```python
from build123d import *

# Parameters (mm, degrees)
SKETCH1_W           = 184.64
SKETCH1_H           = 137
SKETCH1_R           = 3.65
SKETCH1_R_2         = 3.57
SKETCH1_R_3         = 2.5
BOSS_EXTRUDE1_DEPTH = 4
SKETCH3_W           = 104.64
SKETCH3_H           = 20
BOSS_EXTRUDE2_DEPTH = 4
SKETCH6_R           = 3.65
CUT_EXTRUDE4_DEPTH  = 5
SKETCH8_W           = 140
SKETCH8_H           = 16
CUT_EXTRUDE6_DEPTH  = 10
FILLET5_R           = 2
SKETCH11_W          = 184.64
SKETCH11_H          = 15
SKETCH11_R          = 2.5
BOSS_EXTRUDE4_DEPTH = 4
SKETCH12_R          = 2.5
CUT_EXTRUDE8_DEPTH  = 5
SKETCH13_R          = 2.5
CUT_EXTRUDE9_DEPTH  = 10
SKETCH14_W          = 1.5
SKETCH14_H          = 3
CUT_EXTRUDE10_DEPTH = 5


with BuildPart() as part:
    # Sketch1 → Boss-Extrude1 (new body)
    with BuildSketch(Plane.XY):
        with Locations((92.32, 68.5)):
            Rectangle(SKETCH1_W, SKETCH1_H)
        with Locations((15, 16)):
            Circle(SKETCH1_R, mode=Mode.SUBTRACT)
        with Locations((169.64, 16)):
            Circle(SKETCH1_R, mode=Mode.SUBTRACT)
        with Locations((15, 121)):
            Circle(SKETCH1_R_2, mode=Mode.SUBTRACT)
        with Locations((30, 96)):
            Circle(SKETCH1_R_3, mode=Mode.SUBTRACT)
        with Locations((169.64, 121)):
            Circle(SKETCH1_R_2, mode=Mode.SUBTRACT)
        with Locations((154.64, 96)):
            Circle(SKETCH1_R_3, mode=Mode.SUBTRACT)
        Polygon((40, 106), (40, 86), (22.32, 86), (22.32, 56), (162.32, 56), (162.32, 86), (144.64, 86), (144.64, 106), align=None, mode=Mode.SUBTRACT)
    extrude(amount=BOSS_EXTRUDE1_DEPTH)

    # Sketch3 → Boss-Extrude2 (add)
    with BuildSketch(Plane.XY.offset(4)):
        with Locations((92.32, 96)):
            Rectangle(SKETCH3_W, SKETCH3_H)
    extrude(amount=-BOSS_EXTRUDE2_DEPTH)

    # Sketch6 → Cut-Extrude4 (cut, through all)
    with BuildSketch(Plane.XY.offset(4)):
        with Locations((67.32, 16)):
            Circle(SKETCH6_R)
        with Locations((117.32, 16)):
            Circle(SKETCH6_R)
    extrude(amount=-CUT_EXTRUDE4_DEPTH, mode=Mode.SUBTRACT)

    # Sketch8 → Cut-Extrude6 (cut)
    with BuildSketch(Plane.XY.offset(4)):
        with Locations((92.32, 48)):
            Rectangle(SKETCH8_W, SKETCH8_H)
    extrude(amount=-CUT_EXTRUDE6_DEPTH, mode=Mode.SUBTRACT)

    # Fillet5
    fillet5_edges = [part.edges().sort_by_distance(p)[0] for p in [
        (0, 137, 2),
        (184.64, 137, 2),
        (184.64, 0, 2),
        (0, 0, 2),
    ]]
    fillet(fillet5_edges, radius=FILLET5_R)

    # Sketch11 → Boss-Extrude4 (add, through all)
    with BuildSketch(Plane.XY.offset(4)):
        with Locations((92.32, 16)):
            Rectangle(SKETCH11_W, SKETCH11_H)
        with Locations((15, 16)):
            Circle(SKETCH11_R, mode=Mode.SUBTRACT)
        with Locations((169.64, 16)):
            Circle(SKETCH11_R, mode=Mode.SUBTRACT)
    extrude(amount=-BOSS_EXTRUDE4_DEPTH)

    # Sketch12 → Cut-Extrude8 (cut, through all)
    with BuildSketch(Plane.XY.offset(4)):
        with Locations((10, 96)):
            Circle(SKETCH12_R)
        with Locations((174.64, 96)):
            Circle(SKETCH12_R)
    extrude(amount=-CUT_EXTRUDE8_DEPTH, mode=Mode.SUBTRACT)

    # Sketch13 → Cut-Extrude9 (cut)
    with BuildSketch(Plane.XY.offset(4)):
        with Locations((173.48, 67)):
            Circle(SKETCH13_R)
    extrude(amount=-CUT_EXTRUDE9_DEPTH, mode=Mode.SUBTRACT)

    # Sketch14 → Cut-Extrude10 (cut, through all)
    with BuildSketch(Plane.XY.offset(4)):
        with Locations((171.48, 59)):
            Rectangle(SKETCH14_W, SKETCH14_H)
        with Locations((175.48, 59)):
            Rectangle(SKETCH14_W, SKETCH14_H)
    extrude(amount=-CUT_EXTRUDE10_DEPTH, mode=Mode.SUBTRACT)


solid = part.part
```
Build history of the part. All positions in model axes, mm. A direction names the side the tool comes from. Coordinates: 2 decimals unless noted, no trailing zeros. Order: outer loops, then holes, each group sorted by start corner. A loop starts at its lowest first (then second) coordinate and runs counter-clockwise, first axis right, second up. Notation, with made-up numbers: (77.25, 13.25) -> (107.25, 13.25) arc R19 cw to (107.25, 42.25) -> close; hole circle Ø9 at (-9.5, -39.75). An arc over 180 degrees is marked (long way). Answer in a Markdown table with one row per item. Add a question column.
Q1. Band-saw the part on B-B, the plane x = 154.64. List the corners of the cut face in (y, z).
Q2. Drop flat-ended pins along their axis: pin 1 (8 mm diameter, centred on x = 15, y = 121, fed in from +Z); pin 2 (4 mm diameter, centred on x = 169.64, y = 16, fed in from -Z). Give the stop position or say it passes through.
Q3. Band-saw the part on C-C, the plane y = 47.5. List the corners of the cut face in (x, z).
Q4. Wall check: line 1 along X through (y, z) = (58, 1.3); line 2 along Y through (x, z) = (15, 2.6); line 3 along Y through (x, z) = (102.5, 0.2). Give the ranges that are in metal, low to high. Write a range as [from, to].
Q5. Mould opens along X. For faces 1 (the face through (9.67, 98.48, 2.03)), 2 (the face through (172.142, 96.11, 2.028)), 3 (the face through (184.64, 68, 2)), 4 (the face through (0, 68, 2)) say: +X half, -X half, draft (parallel to the pull), parting line (faces both ways), or undercut.
Q6. Band-saw the part on A-A, the plane y = 16. List the corners of the cut face in (x, z).
Q7. Band-saw the part on D-D, the plane z = 1.8. Give the number of separate pieces and of enclosed holes in the cut face, then the cut area to 3 significant figures.
Q8. Which spindle directions (+Z, -Z, +X, -X, +Y, -Y) get a long thin tool onto all of the face, cutting with end or side? Do faces 5 (the face through (91, 40, 2)), 6 (the face through (91, 0, 2)). Say none if no direction does.
Answers follow:
| question | item | result |
|---|---|---|
| 1 | outline | (0, 0) -> (40, 0) -> (40, 4) -> (0, 4) -> close; (86, 0) -> (93.5, 0) -> (93.5, 4) -> (86, 4) -> close; (98.5, 0) -> (137, 0) -> (137, 4) -> (98.5, 4) -> close |
| 2 | pin 1 | z = 4 |
| 2 | pin 2 | through |
| 3 | outline | (0, 0) -> (22.32, 0) -> (22.32, 4) -> (0, 4) -> close; (162.32, 0) -> (184.64, 0) -> (184.64, 4) -> (162.32, 4) -> close |
| 4 | line 1 | [0, 22.32], [162.32, 170.73], [172.23, 174.73], [176.23, 184.64] |
| 4 | line 2 | [0, 13.5], [18.5, 117.43], [124.57, 137] |
| 4 | line 3 | [0, 40], [86, 137] |
| 5 | face 1 | undercut |
| 5 | face 2 | undercut |
| 5 | face 3 | +X half |
| 5 | face 4 | -X half |
| 6 | outline | (0, 0) -> (12.5, 0) -> (12.5, 4) -> (0, 4) -> close; (17.5, 0) -> (167.14, 0) -> (167.14, 4) -> (17.5, 4) -> close; (172.14, 0) -> (184.64, 0) -> (184.64, 4) -> (172.14, 4) -> close |
| 7 | separate pieces | 1 |
| 7 | enclosed holes | 12 |
| 7 | area | 18,600 mm^2 |
| 8 | face 5 | +Z, -Z |
| 8 | face 6 | +Z, -Z, +X, -X, -Y |
